Verification items for the finished model (mm, model axes). Round coordinates to 2 decimals unless told otherwise and drop trailing zeros. Order: outer loops, then holes, each group sorted by start corner. A loop starts at its lowest first (then second) coordinate and runs counter-clockwise, first axis right, second up. Notation, with made-up numbers: M -14.5,-33 L 9.5,-33 A14 cw 9.5,-15 Z; hole C -14,-8 d8. An arc over 180 degrees is marked long. Answer as a JSON object with one key per item and string values. Group by question number.
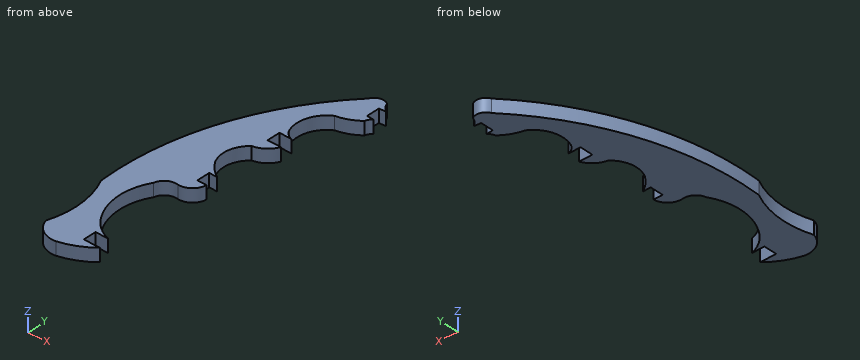
```python
from build123d import *

# Parameters (mm, degrees)
BOSS_EXTRUDE1_DEPTH = 1.524


with BuildPart() as part:
    # Sketch1 → Boss-Extrude1 (new body)
    with BuildSketch(Plane.XY):
        with BuildLine():
            Line((-110.824360774, 0), (-110.824360774, -1.524))
            Line((-110.824360774, -1.524), (-108.927743626, -1.524))
            ThreePointArc((-108.927743626, -1.524), (-110.568786986, -2.659932295), (-112.442883949, -3.346318527))
            ThreePointArc((-112.442883949, -3.346318527), (-114.17716098, -2.968961004), (-115.207793415, -1.524))
            ThreePointArc((-115.207793415, -1.524), (-114.703070876, 2.396926331), (-115.749307819, 6.209247985))
            ThreePointArc((-115.749307819, 6.209247985), (-113.92263745, 19.565030778), (-106.916865485, 31.081663004))
            ThreePointArc((-106.916865485, 31.081663004), (-106.184950927, 31.736506317), (-105.211200263, 31.608723968))
            ThreePointArc((-105.211200263, 31.608723968), (-104.901513118, 31.0579276), (-104.454303839, 30.611512291))
            Line((-104.454303839, 30.611512291), (-105.211200263, 30.544825407))
            Line((-105.211200263, 30.544825407), (-105.211200263, 29.025368505))
            Line((-105.211200263, 29.025368505), (-104.403994808, 28.977437337))
            ThreePointArc((-104.403994808, 28.977437337), (-104.700603167, 28.683060455), (-104.849681876, 28.292663471))
            ThreePointArc((-104.849681876, 28.292663471), (-106.016123504, 27.550057971), (-107.333979522, 27.131364149))
            ThreePointArc((-107.333979522, 27.131364149), (-108.818673483, 25.32832607), (-108.817338403, 22.992676119))
            ThreePointArc((-108.817338403, 22.992676119), (-108.405188947, 22.369705182), (-107.752531072, 22.00639036))
            Line((-107.752531072, 22.00639036), (-109.139263732, 22.00639036))
            Line((-109.139263732, 22.00639036), (-109.139263732, 20.478701595))
            Line((-109.139263732, 20.478701595), (-107.557691458, 20.478701595))
            ThreePointArc((-107.557691458, 20.478701595), (-108.363599409, 19.419942847), (-109.579185571, 18.87882549))
            ThreePointArc((-109.579185571, 18.87882549), (-110.645223511, 17.073742216), (-110.328866367, 15.001381081))
            ThreePointArc((-110.328866367, 15.001381081), (-109.579185571, 14.069438674), (-108.625140976, 13.348094888))
            Line((-108.625140976, 13.348094888), (-109.551135599, 13.348094888))
            Line((-109.551135599, 13.348094888), (-109.551135599, 11.811176348))
            Line((-109.551135599, 11.811176348), (-108.478697007, 11.811176348))
            ThreePointArc((-108.478697007, 11.811176348), (-109.071957304, 10.623612067), (-110.328866367, 10.196474724))
            ThreePointArc((-110.328866367, 10.196474724), (-111.484723908, 9.970154225), (-112.1438695, 8.994062677))
            ThreePointArc((-112.1438695, 8.994062677), (-113.066844869, 5.45696931), (-111.950245848, 1.976147619))
            ThreePointArc((-111.950245848, 1.976147619), (-110.838027473, 0.758299628), (-109.373389254, 0))
            Line((-109.373389254, 0), (-110.824360774, 0))
        make_face()
    extrude(amount=BOSS_EXTRUDE1_DEPTH)


solid = part.part
```
Q1. Cross-section at B-B, the plane x = -114. Record the cut outline in (y, z).
Q2. Cross-section at C-C, the plane y = 16.5. Record the cut outline in (x, z), then the cut area to 3 significant figures.
Q3. Gauge pin test, flat ends, axial feed: pin 1 Ø0.5 at (y, z) = (21.5, 0.5) entering from +X; pin 2 Ø0.5 at (x, z) = (-110, 1) entering from +Y; pin 3 Ø2 at (x, y) = (-113, 25.5) entering from -Z; pin 4 Ø0.5 at (x, z) = (-108.5, 1) entering from +Y. Record the tip position at first contact, or that the pin passes through.
Q4. Thickness scan on line 1 (Y direction, x = -110.25, z = 0.3); line 2 (Y direction, x = -110.75, z = 0.1); line 3 (Y direction, x = -108.25, z = 0.3). Record the ranges inside material, lowest first. Write a range as from..to.
Conclusion:
{
 "1": {"outline": "M -3.08,0 L 19.34,0 L 19.34,1.52 L -3.08,1.52 Z"},
 "2": {"outline": "M -114.85,0 L -110.7,0 L -110.7,1.52 L -114.85,1.52 Z", "area": "6.32 mm2"},
 "3": {"pin 1": "x = -109.14", "pin 2": "y = 27.61", "pin 3": "through", "pin 4": "y = 29.57"},
 "4": {"line 1": "-2.49..-1.52, 0..0.37, 10.19..14.88, 18.1..26.88", "line 2": "-2.75..-1.52, 0..0.69, 10.22..26.11", "line 3": "19.52..20.48, 22.01..22.24, 26.34..29.57"}
}
